from build123d import *

# Parameters (mm, degrees)
EXTRUDE_1_DEPTH = 4.3


with BuildPart() as part:
    # 草图1 → 凸台-拉伸1 (new body)
    with BuildSketch(Plane.XY):
        Polygon((31.812419505, -35.7), (31.812419505, -40), (3, -40), (3, -35.7), (3, 0), (31.812419505, 0), align=None)
        with BuildLine():
            Line((20.928372126, -7.487592169), (20.928372126, -28.212407831))
            ThreePointArc((20.928372126, -28.212407831), (17.406209752, -31.734570205), (13.884047379, -28.212407831))
            Line((13.884047379, -28.212407831), (13.884047379, -7.487592169))
            ThreePointArc((13.884047379, -7.487592169), (17.406209752, -3.965429795), (20.928372126, -7.487592169))
        make_face(mode=Mode.SUBTRACT)
    extrude(amount=EXTRUDE_1_DEPTH)


solid = part.part
Check sheet for the modelled part. Datum: model origin and axes. Units: mm. A direction names the side the tool comes from. Round coordinates to 2 decimals unless told otherwise and drop trailing zeros. Loops run counter-clockwise (first coordinate to the right, second up) from the corner with the lowest first, then second, coordinate; pieces in that order, holes last.
1. Sectioned sample at A-A on y = -15. Record the boundary of the cut face in (x, z).
2. Sectioned sample at C-C on z = 0.4. Record the boundary of the cut face in (x, y).
3. Mould release check, pull along Y, two halves, no side actions. Record for faces 3 (the cylindrical face through (17.484, -31.734, 2.12)), 4 (the flat face through (17, 0, 2)), 5 (the flat face through (3, -20, 2)): released by +Y, released by -Y, zero draft, split by the parting line, or undercut.
4. Sectioned sample at B-B on x = 15.25. Record the boundary of the cut face in (y, z), and give its area (3 significant figures).
5. Set-up check for faces 1 (the flat face through (24, -20, 0)), 2 (the flat face through (13.884, -18, 2)): record each of +Z, -Z, +X, -X, +Y, -Y from which the full face is reachable in a straight line by a thin tool's end or side.
6. Scan lines: probe 1 along X at (y, z) = (-18, 3.3); probe 2 along Y at (x, z) = (15, 0.65); probe 3 along X at (y, z) = (-30, 1.6). Record each from-to range of solid material in increasing order.
Recorded:
1. outline: (3, 0) - (13.88, 0) - (13.88, 4.3) - (3, 4.3) - close; (20.93, 0) - (31.81, 0) - (31.81, 4.3) - (20.93, 4.3) - close
2. outline: (3, -40) - (31.81, -40) - (31.81, 0) - (3, 0) - close; hole (13.88, -28.21) arc R3.52 ccw to (20.93, -28.21) - (20.93, -7.49) arc R3.52 ccw to (13.88, -7.49) - close
3. face 3: undercut
3. face 4: released by +Y
3. face 5: zero draft
4. outline: (-40, 0) - (-31, 0) - (-31, 4.3) - (-40, 4.3) - close; (-4.7, 0) - (0, 0) - (0, 4.3) - (-4.7, 4.3) - close
4. area: 58.9 mm2
5. face 1: -Z, +X, -X, +Y, -Y
5. face 2: +Z, -Z
6. probe 1: x = 3 to 13.88, 20.93 to 31.81
6. probe 2: y = -40 to -30.78, -4.92 to 0
6. probe 3: x = 3 to 14.37, 20.44 to 31.81
